```python
from build123d import *

# Parameters (mm, degrees)
F0_W     = 27
F0_H     = 27
F1_DEPTH = 3
F2_W     = 3
F2_H     = 3
F3_DEPTH = 3
F4_W     = 27
F4_H     = 27
F5_DEPTH = 3
F6_R     = 1


with BuildPart() as f1:
    # F0 (on Front) → F1 (new body)
    with BuildSketch(Plane.XZ):
        Rectangle(F0_W, F0_H)
    extrude(amount=F1_DEPTH)

    # F2 (on face) → F3 (join)
    with BuildSketch(Plane.XZ.offset(3)):
        with Locations((-12, 12)):
            Rectangle(F2_W, F2_H)
        with Locations((12, 12)):
            Rectangle(F2_W, F2_H)
        with Locations((12, -12)):
            Rectangle(F2_W, F2_H)
        with Locations((-12, -12)):
            Rectangle(F2_W, F2_H)
    extrude(amount=F3_DEPTH)

    # F4 (on face) → F5 (join)
    with BuildSketch(Plane.XZ.offset(6)):
        Rectangle(F4_W, F4_H)
    extrude(amount=F5_DEPTH)

    # F6
    f6_edges = [f1.edges().sort_by_distance(p)[0] for p in [
        (-13.5, -9, 0),
        (0, -9, 13.5),
        (13.5, -9, 0),
        (0, -9, -13.5),
        (-13.5, -3, 0),
        (-13.5, -6, 0),
        (-13.5, -4.5, 10.5),
        (-13.5, -4.5, -10.5),
        (0, -6, -13.5),
        (-10.5, -4.5, -13.5),
        (0, -3, -13.5),
        (10.5, -4.5, -13.5),
        (13.5, -4.5, -10.5),
        (13.5, -6, 0),
        (13.5, -4.5, 10.5),
        (13.5, -3, 0),
        (10.5, -4.5, 13.5),
        (0, -6, 13.5),
        (-10.5, -4.5, 13.5),
        (0, -3, 13.5),
        (10.5, -4.5, 10.5),
        (10.5, -4.5, -10.5),
        (-10.5, -4.5, -10.5),
        (-10.5, -4.5, 10.5),
        (-13.5, -4.5, 13.5),
        (13.5, -4.5, 13.5),
        (13.5, -4.5, -13.5),
        (-13.5, -4.5, -13.5),
    ]]
    fillet(f6_edges, radius=F6_R)


solid = f1.part
```
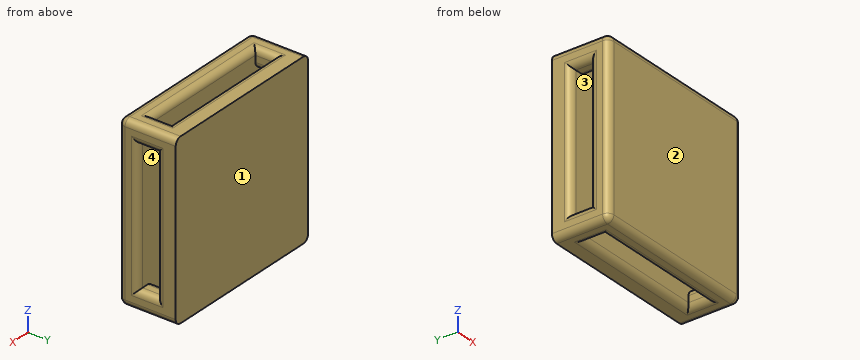
Design review of the part built by this model. Coordinates are the model's own, in mm. Face numbers are marked on the shaded views. Round coordinates to 2 decimals unless told otherwise and drop trailing zeros. Write each loop counter-clockwise with the first axis right and the second up, starting at its lowest first coordinate (ties: lowest second). Pieces come first, ordered by that corner, then holes.
Item 1: The part is to be moulded in two halves that separate along Y. For the marked faces 1, 2, 3 and 4, say which applies: +Y half, -Y half, draft (parallel to the pull), parting line (faces both ways), or undercut.
Item 2: We need section C-C on x = -4. Write out the cut boundary in (y, z).
Item 3: We need section D-D on x = -11. Write out the cut boundary in (y, z).
Item 4: We need section B-B on z = -10. Write out the cut boundary in (x, y), and give its area (3 significant figures).
Item 5: We need section A-A on y = -5.25. State how many separate pieces and enclosed holes the cut face has, and give its area (3 significant figures).
Item 6: Clearance check with a flat-ended pin moving along its axis: pin 1 Ø2 at (x, z) = (7, 9.5) entering from +Y. State where the tip first meets the part, or that it passes through.
Item 7: For probe 1 along Y at (x, z) = (0.75, 6.75); probe 2 along X at (y, z) = (-4.25, 11.75); probe 3 along Z at (x, y) = (-10.75, -5.5), list the stretches that pass through material, from the lowest coordinate up.
Returned:
1. face 1: +Y half
1. face 2: -Y half
1. face 3: undercut
1. face 4: undercut
2. outline: (-9, -12.5) arc R1 ccw to (-8, -13.5) - (-7, -13.5) arc R1 ccw to (-6, -12.5) - (-6, 12.5) arc R1 ccw to (-7, 13.5) - (-8, 13.5) arc R1 ccw to (-9, 12.5) - close; (-3, -12.5) arc R1 ccw to (-2, -13.5) - (0, -13.5) - (0, 13.5) - (-2, 13.5) arc R1 ccw to (-3, 12.5) - close
3. outline: (-9, -12.5) arc R1 ccw to (-8, -13.5) - (-7, -13.5) arc R1 ccw to (-6.5, -13.37) - (-2.5, -13.37) arc R1 ccw to (-2, -13.5) - (0, -13.5) - (0, 13.5) - (-2, 13.5) arc R1 ccw to (-2.5, 13.37) - (-6.5, 13.37) arc R1 ccw to (-7, 13.5) - (-8, 13.5) arc R1 ccw to (-9, 12.5) - close; hole (-6, -10.63) - (-3, -10.63) - (-3, 10.63) - (-6, 10.63) - close
4. outline: (-13.5, -8) arc R1 ccw to (-12.5, -9) - (12.5, -9) arc R1 ccw to (13.5, -8) - (13.5, -7) arc R1 ccw to (12.5, -6) - (-12.5, -6) arc R1 ccw to (-13.5, -7) - close; (-13.5, -2) arc R1 ccw to (-12.5, -3) - (12.5, -3) arc R1 ccw to (13.5, -2) - (13.5, 0) - (-13.5, 0) - close
4. area: 161 mm2
5. separate pieces: 4
5. enclosed holes: 0
5. area: 32.6 mm2
6. pin 1: stops at y = 0
7. probe 1: y = -9 to -6, -3 to 0
7. probe 2: x = -13.5 to -10.5, 10.5 to 13.5
7. probe 3: z = -13.16 to -10.84, 10.84 to 13.16
